Build history of the part. All positions in model axes, mm. Face numbers are marked on the shaded views. A direction names the side the tool comes from. Give positions to 0.01 mm unless a question says otherwise; leave off trailing zeros. Order: outer loops, then holes, each group sorted by start corner. A loop starts at its lowest first (then second) coordinate and runs counter-clockwise, first axis right, second up. Notation, with made-up numbers: (36.5, 57.25) - (68.5, 57.25) arc R5 cw to (68.5, 61.25) - close; hole circle Ø7 at (-5.75, 26). An arc over 180 degrees is marked (long way). Answer in a Markdown table with one row per item.
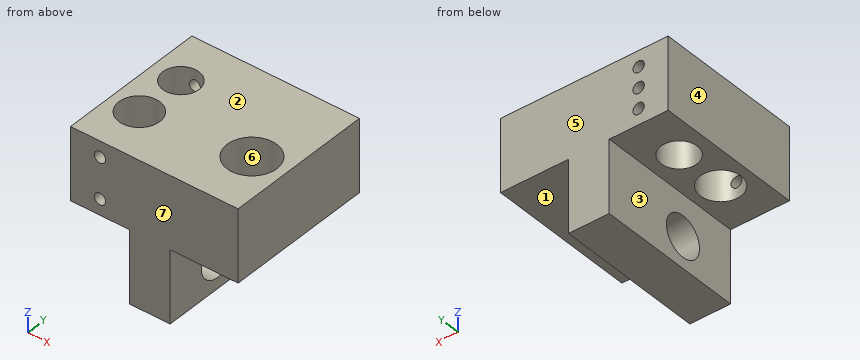
```python
from build123d import *

# Parameters (mm, degrees)
ESQUISSE1_W             = 37
ESQUISSE1_H             = 16
BOSS_EXTRU_1_DEPTH      = 16.5
ESQUISSE3_R             = 5.5
ENL_V_MAT_EXTRU_2_DEPTH = 30.504236984
ESQUISSE14_R            = 4.5
ENL_V_MAT_EXTRU_3_DEPTH = 30.504236984
ESQUISSE15_R            = 4
ENL_V_MAT_EXTRU_4_DEPTH = 30.504236984
TROU_TARAUD_M34_REACH   = 40.668
TROU_TARAUD_M34_BORE_R  = 1.25
TROU_TARAUD_M35_REACH   = 40.668
TROU_TARAUD_M35_BORE_R  = 1.25
TROU_TARAUD_M36_REACH   = 41.444
TROU_TARAUD_M36_BORE_R  = 1.25
ESQUISSE18_W            = 9
ESQUISSE18_H            = 16
BOSS_EXTRU_2_DEPTH      = 33
ESQUISSE20_R            = 4.5
ENL_V_MAT_EXTRU_5_DEPTH = 38.73923692


with BuildPart() as part:
    # Esquisse1 → Boss.-Extru.1 (new, symmetric)
    with BuildSketch(Plane(origin=(0, 0, 0), x_dir=(1, 0, 0), z_dir=(0, 1, 0))):
        Rectangle(ESQUISSE1_W, ESQUISSE1_H)
    extrude(amount=BOSS_EXTRU_1_DEPTH, both=True)

    # Esquisse3 → Enlèv. mat.-Extru.2 (cut, through all)
    with BuildSketch(Plane.XY.offset(8)):
        with Locations((11, -3.5)):
            Circle(ESQUISSE3_R)
    extrude(amount=-ENL_V_MAT_EXTRU_2_DEPTH, mode=Mode.SUBTRACT)

    # Esquisse14 → Enlèv. mat.-Extru.3 (cut, through all)
    with BuildSketch(Plane(origin=(0, 0, -8), x_dir=(-1, 0, 0), z_dir=(0, 0, -1))):
        with Locations((12, -5.8)):
            Circle(ESQUISSE14_R)
    extrude(amount=-ENL_V_MAT_EXTRU_3_DEPTH, mode=Mode.SUBTRACT)

    # Esquisse15 → Enlèv. mat.-Extru.4 (cut, through all)
    with BuildSketch(Plane(origin=(0, 0, -8), x_dir=(-1, 0, 0), z_dir=(0, 0, -1))):
        with Locations((12, 5.5)):
            Circle(ESQUISSE15_R)
    extrude(amount=-ENL_V_MAT_EXTRU_4_DEPTH, mode=Mode.SUBTRACT)

    # Trou taraudé M34 bore → Trou taraudé M34 (cut, up to next)
    with BuildSketch(Plane(origin=(0, 16.5, 0), x_dir=(1, 0, 0), z_dir=(0, 1, 0)), mode=Mode.PRIVATE) as trou_taraud_m34_sk1:
        with Locations((-12, -4.5)):
            Circle(TROU_TARAUD_M34_BORE_R)
    trou_taraud_m34_tool1 = extrude(trou_taraud_m34_sk1.sketch, amount=-TROU_TARAUD_M34_REACH, mode=Mode.PRIVATE) & part.part
    # Trou taraudé M34 bore → Trou taraudé M34 (cut, up to next)
    with BuildSketch(Plane(origin=(0, 16.5, 0), x_dir=(1, 0, 0), z_dir=(0, 1, 0)), mode=Mode.PRIVATE) as trou_taraud_m34_sk2:
        with Locations((-12, 4.5)):
            Circle(TROU_TARAUD_M34_BORE_R)
    trou_taraud_m34_tool2 = extrude(trou_taraud_m34_sk2.sketch, amount=-TROU_TARAUD_M34_REACH, mode=Mode.PRIVATE) & part.part
    add(trou_taraud_m34_tool1.solids().sort_by_distance((-12, 16.5, 4.5))[0], mode=Mode.SUBTRACT)
    add(trou_taraud_m34_tool2.solids().sort_by_distance((-12, 16.5, -4.5))[0], mode=Mode.SUBTRACT)

    # Trou taraudé M35 bore → Trou taraudé M35 (cut, up to next)
    with BuildSketch(Plane(origin=(0, -16.5, 0), x_dir=(-1, 0, 0), z_dir=(0, -1, 0)), mode=Mode.PRIVATE) as trou_taraud_m35_sk1:
        with Locations((12, -4.5)):
            Circle(TROU_TARAUD_M35_BORE_R)
    trou_taraud_m35_tool1 = extrude(trou_taraud_m35_sk1.sketch, amount=-TROU_TARAUD_M35_REACH, mode=Mode.PRIVATE) & part.part
    # Trou taraudé M35 bore → Trou taraudé M35 (cut, up to next)
    with BuildSketch(Plane(origin=(0, -16.5, 0), x_dir=(-1, 0, 0), z_dir=(0, -1, 0)), mode=Mode.PRIVATE) as trou_taraud_m35_sk2:
        with Locations((12, 4.5)):
            Circle(TROU_TARAUD_M35_BORE_R)
    trou_taraud_m35_tool2 = extrude(trou_taraud_m35_sk2.sketch, amount=-TROU_TARAUD_M35_REACH, mode=Mode.PRIVATE) & part.part
    add(trou_taraud_m35_tool1.solids().sort_by_distance((-12, -16.5, 4.5))[0], mode=Mode.SUBTRACT)
    add(trou_taraud_m35_tool2.solids().sort_by_distance((-12, -16.5, -4.5))[0], mode=Mode.SUBTRACT)

    # Trou taraudé M36 bore → Trou taraudé M36 (cut, up to next)
    with BuildSketch(Plane(origin=(-1.446004376, 16.5, -0.30351444), x_dir=(-1, 0, 0), z_dir=(0, 1, 0)), mode=Mode.PRIVATE) as trou_taraud_m36_sk1:
        with Locations((10.553995624, 0.30351444)):
            Circle(TROU_TARAUD_M36_BORE_R)
    trou_taraud_m36_tool1 = extrude(trou_taraud_m36_sk1.sketch, amount=-TROU_TARAUD_M36_REACH, mode=Mode.PRIVATE) & part.part
    add(trou_taraud_m36_tool1.solids().sort_by_distance((-12, 16.5, 0))[0], mode=Mode.SUBTRACT)

    # Esquisse18 → Boss.-Extru.2 (add)
    with BuildSketch(Plane.XZ.offset(16.5)):
        with Locations((-1, -16)):
            Rectangle(ESQUISSE18_W, ESQUISSE18_H)
    extrude(amount=-BOSS_EXTRU_2_DEPTH)

    # Esquisse20 → Enlèv. mat.-Extru.5 (cut, through all)
    with BuildSketch(Plane.ZY.offset(5.5)):
        with Locations((-17.1, -3.55)):
            Circle(ESQUISSE20_R)
    extrude(amount=-ENL_V_MAT_EXTRU_5_DEPTH, mode=Mode.SUBTRACT)


solid = part.part
```
1. Which spindle directions (+Z, -Z, +X, -X, +Y, -Y) get a long thin tool onto all of the face, cutting with end or side? Do the marked faces 1, 2 and 3. Say none if no direction does.
Check result:
| item | result |
|---|---|
| face 1 | -Z, +X, +Y, -Y |
| face 2 | +Z, +X, -X, +Y, -Y |
| face 3 | -Z, -X, +Y, -Y |
2. Probe line 1 (Y direction, x = -12, z = -2); line 2 (Z direction, x = -12, y = 12); line 3 (Z direction, x = -12, y = -13). List the from-to ranges inside material, lowest first.
Check result:
| item | result |
|---|---|
| line 1 | y = -16.5 to -10.3, -1.3 to 1.5, 9.5 to 16.5 |
| line 2 | z = -8 to -5.75, -3.25 to -1.25, 1.25 to 3.25, 5.75 to 8 |
| line 3 | z = -8 to -5.75, -3.25 to 3.25, 5.75 to 8 |
3. Two-plate mould, pull along Y, no slides. Class the marked faces 4, 5, 6 and 7: +Y half, -Y half, draft (parallel to the pull), parting line (faces both ways), or undercut.
Check result:
| item | result |
|---|---|
| face 4 | draft |
| face 5 | +Y half |
| face 6 | undercut |
| face 7 | -Y half |
4. Cut at B-B on z = 6.5. Write the cut outline in (x, y).
Check result:
| item | result |
|---|---|
| outline | (-18.5, -16.5) - (18.5, -16.5) - (18.5, 16.5) - (-18.5, 16.5) - close; hole circle Ø9 at (-12, -5.8); hole circle Ø8 at (-12, 5.5); hole circle Ø11 at (11, -3.5) |
5. Cut at C-C on x = -12. Count the separate pieces of the cut face and the enclosed holes in it, and give its area (4 significant figures).
Check result:
| item | result |
|---|---|
| separate pieces | 8 |
| enclosed holes | 0 |
| area | 172.5 mm² |
6. Cut at D-D on z = 0. Write the cut outline in (x, y).
Check result:
| item | result |
|---|---|
| outline | (-18.5, -16.5) - (18.5, -16.5) - (18.5, 16.5) - (-10.75, 16.5) - (-10.75, 9.3) arc R4 cw (long way) to (-13.25, 9.3) - (-13.25, 16.5) - (-18.5, 16.5) - close; hole circle Ø9 at (-12, -5.8); hole circle Ø11 at (11, -3.5) |
7. Cut at A-A on x = 11. Write the cut outline in (y, z).
Check result:
| item | result |
|---|---|
| outline | (-16.5, -8) - (-9, -8) - (-9, 8) - (-16.5, 8) - close; (2, -8) - (16.5, -8) - (16.5, 8) - (2, 8) - close |
8. Drop flat-ended pins along their axis: P1, Ø5, axis at y = -7, z = -19.5, coming from the +X side; P2, Ø1.5, axis at x = -12, z = 4.5, coming from the +Y side; P3, Ø14.5, axis at x = -9, y = 1.5, coming from the -Z side; P4, Ø9, axis at x = -12, y = 5.5, coming from the -Z side. Give the stop position or say it passes through.
Check result:
| item | result |
|---|---|
| P1 | stops at x = 3.5 |
| P2 | stops at y = 1.57 |
| P3 | stops at z = -24 |
| P4 | stops at z = -8 |
